Input: part model. Units: mm. Frame: model coordinates. Face numbers are marked on the shaded views. Round coordinates to 2 decimals unless told otherwise and drop trailing zeros. Loops run counter-clockwise (first coordinate to the right, second up) from the corner with the lowest first, then second, coordinate; pieces in that order, holes last.
(1) First-contact query: pin 1 Ø2 at (x, z) = (-11.5, 0) entering from -Y (3 decimals). Flat tip, straight axial feed; report the tip coordinate or a pass-through.
(2) Draft query along Z for the marked faces 1, 2, 3 and 4. Return one class per face: released by +Z, released by -Z, zero draft, split by the parting line, or undercut.
(3) Line query: line 1 (X direction, y = 0.8, z = 0); line 2 (X direction, y = 2.7, z = 0.75); line 3 (Z direction, x = -5.5, y = 2.75). Output: solid intervals per line, ascending.
(4) Cut plane A-A, the plane y = 1.85. Output: boundary loops of the cut face in (x, z), and give its area (3 significant figures).
(5) Cut plane C-C, the plane x = 0. Output: boundary loops of the cut face in (y, z).
(6) Cut plane B-B, the plane z = 0. Output: boundary loops of the cut face in (x, y).
(7) Cut plane D-D, the plane z = 2.5. Output: boundary loops of the cut face in (x, y).
from build123d import *

# Parameters (mm, degrees)
SKETCH1_R           = 3.75
SKETCH1_R_2         = 1.25
SKETCH1_R_3         = 1
BOSS_EXTRUDE1_DEPTH = 3
FILLET1_R           = 1.5


with BuildPart() as part:
    # Sketch1 → Boss-Extrude1 (new body)
    with BuildSketch(Plane(origin=(0, 0, 0), x_dir=(1, 0, 0), z_dir=(0, 1, 0))):
        with BuildLine():
            Line((-2.277845841, 4.451001946), (-13.5, 2))
            Line((-13.5, 2), (-13.5, -2))
            Line((-13.5, -2), (-2.277845841, -4.451001946))
            ThreePointArc((-2.277845841, -4.451001946), (0, -5), (2.277845841, -4.451001946))
            Line((2.277845841, -4.451001946), (13.5, -2))
            Line((13.5, -2), (13.5, 2))
            Line((13.5, 2), (2.277845841, 4.451001946))
            ThreePointArc((2.277845841, 4.451001946), (0, 5), (-2.277845841, 4.451001946))
        make_face()
        Circle(SKETCH1_R, mode=Mode.SUBTRACT)
        with Locations((-11.5, 0)):
            Circle(SKETCH1_R_2, mode=Mode.SUBTRACT)
        with Locations((11.5, 0)):
            Circle(SKETCH1_R_2, mode=Mode.SUBTRACT)
        with Locations((-7, 0)):
            Circle(SKETCH1_R_3, mode=Mode.SUBTRACT)
    extrude(amount=BOSS_EXTRUDE1_DEPTH)

    # Fillet1
    fillet1_edges = [part.edges().sort_by_distance(p)[0] for p in [
        (-13.5, 1.5, 2),
        (-13.5, 1.5, -2),
        (13.5, 1.5, -2),
        (13.5, 1.5, 2),
    ]]
    fillet(fillet1_edges, radius=FILLET1_R)


solid = part.part
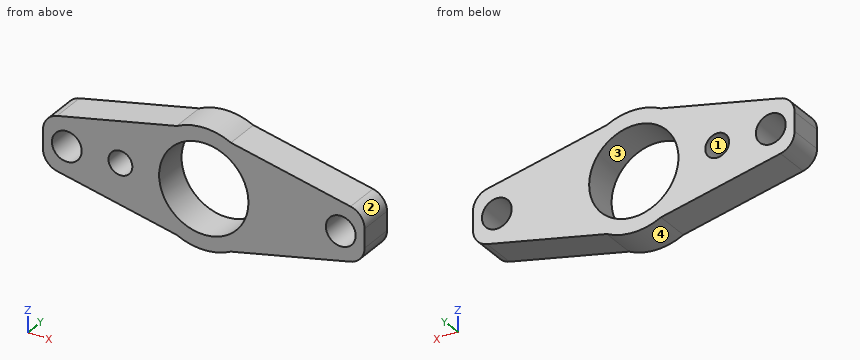
Reported:
1. pin 1: passes through
2. face 1: undercut
2. face 2: released by +Z
2. face 3: undercut
2. face 4: released by -Z
3. line 1: x = -13.5 to -12.75, -10.25 to -8, -6 to -3.75, 3.75 to 10.25, 12.75 to 13.5
3. line 2: x = -13.5 to -12.5, -10.5 to -7.66, -6.34 to -3.67, 3.67 to 10.5, 12.5 to 13.5
3. line 3: z = -3.75 to 3.75
4. outline: (-13.5, -0.79) arc R1.5 ccw to (-12.32, -2.26) - (-2.28, -4.45) arc R5 ccw to (2.28, -4.45) - (12.32, -2.26) arc R1.5 ccw to (13.5, -0.79) - (13.5, 0.79) arc R1.5 ccw to (12.32, 2.26) - (2.28, 4.45) arc R5 ccw to (-2.28, 4.45) - (-12.32, 2.26) arc R1.5 ccw to (-13.5, 0.79) - close; hole circle Ø2.5 at (-11.5, 0); hole circle Ø2 at (-7, 0); hole circle Ø7.5 at (0, 0); hole circle Ø2.5 at (11.5, 0)
4. area: 130 mm2
5. outline: (0, -5) - (3, -5) - (3, -3.75) - (0, -3.75) - close; (0, 3.75) - (3, 3.75) - (3, 5) - (0, 5) - close
6. outline: (-13.5, 0) - (-12.75, 0) - (-12.75, 3) - (-13.5, 3) - close; (-10.25, 0) - (-8, 0) - (-8, 3) - (-10.25, 3) - close; (-6, 0) - (-3.75, 0) - (-3.75, 3) - (-6, 3) - close; (3.75, 0) - (10.25, 0) - (10.25, 3) - (3.75, 3) - close; (12.75, 0) - (13.5, 0) - (13.5, 3) - (12.75, 3) - close
7. outline: (-11.21, 0) - (-2.8, 0) - (-2.8, 3) - (-11.21, 3) - close; (2.8, 0) - (11.21, 0) - (11.21, 3) - (2.8, 3) - close
